from build123d import *

# Parameters (mm, degrees)
SKETCH1_W           = 93.58
SKETCH1_H           = 68.18
BOSS_EXTRUDE1_DEPTH = 5
SKETCH1_12_W        = 73.58
SKETCH1_12_H        = 48.18
CUT_EXTRUDE2_DEPTH  = 59.107075301
FILLET1_R           = 5
FILLET2_R           = 5
SKETCH1_13_R        = 2
CUT_EXTRUDE3_DEPTH  = 59.107075301
SKETCH2_W           = 50.18
SKETCH2_H           = 1.1
CUT_EXTRUDE4_DEPTH  = 88.58


with BuildPart() as part:
    # Sketch1 → Boss-Extrude1 (new body)
    with BuildSketch(Plane(origin=(0, 0, 0), x_dir=(1, 0, 0), z_dir=(0, 1, 0))):
        Rectangle(SKETCH1_W, SKETCH1_H)
    extrude(amount=BOSS_EXTRUDE1_DEPTH)

    # Sketch1<12> → Cut-Extrude2 (cut, through all)
    with BuildSketch(Plane(origin=(0, 0, 0), x_dir=(1, 0, 0), z_dir=(0, 1, 0))):
        Rectangle(SKETCH1_12_W, SKETCH1_12_H)
    extrude(amount=CUT_EXTRUDE2_DEPTH, mode=Mode.SUBTRACT)

    # Fillet1
    fillet1_edges = [part.edges().sort_by_distance(p)[0] for p in [
        (-46.79, 2.5, 34.09),
        (-46.79, 2.5, -34.09),
        (46.79, 2.5, -34.09),
        (46.79, 2.5, 34.09),
    ]]
    fillet(fillet1_edges, radius=FILLET1_R)

    # Fillet2
    fillet2_edges = [part.edges().sort_by_distance(p)[0] for p in [
        (-36.79, 2.5, -24.09),
        (-36.79, 2.5, 24.09),
        (36.79, 2.5, 24.09),
        (36.79, 2.5, -24.09),
    ]]
    fillet(fillet2_edges, radius=FILLET2_R)

    # Sketch1<13> → Cut-Extrude3 (cut, through all)
    with BuildSketch(Plane(origin=(0, 0, 0), x_dir=(1, 0, 0), z_dir=(0, 1, 0))):
        with Locations(Location((-41.79, 29.09, 0), (0, 0, 270))):
            Circle(SKETCH1_13_R)
        with Locations(Location((41.79, 29.09, 0), (0, 0, 90))):
            Circle(SKETCH1_13_R)
        with Locations(Location((41.79, -29.09, 0), (0, 0, 270))):
            Circle(SKETCH1_13_R)
        with Locations(Location((-41.79, -29.09, 0), (0, 0, 90))):
            Circle(SKETCH1_13_R)
    extrude(amount=CUT_EXTRUDE3_DEPTH, mode=Mode.SUBTRACT)

    # Sketch2 → Cut-Extrude4 (cut)
    with BuildSketch(Plane.ZY.offset(46.79)):
        with Locations((0, 2.5)):
            Rectangle(SKETCH2_W, SKETCH2_H)
    extrude(amount=-CUT_EXTRUDE4_DEPTH, mode=Mode.SUBTRACT)


solid = part.part
Part model, mm, in its own coordinate system. A direction names the side the tool comes from. Give positions to 0.01 mm unless a question says otherwise; leave off trailing zeros. Loops run counter-clockwise (first coordinate to the right, second up) from the corner with the lowest first, then second, coordinate; pieces in that order, holes last. Notation, with made-up numbers: M 28,19.5 L 79,19.5 A34 cw 79,51.5 Z; hole C 51,-26.5 d4. An arc over 180 degrees is marked long. Put each result on its own line as item: value. Start each with the question number.
1) Pull direction X, two halves, no side cores. Call faces 3 (the flat face through (-19.1, 3.05, -24.3)), 4 (the cylindrical face through (35.29, 0.99, 22.66)), 5 (the cylindrical face through (-45.36, 2.54, 32.59)), 6 (the cylindrical face through (-43.742, 2.465, -29.524)): +X half, -X half, draft (parallel to the pull), parting line (faces both ways), or undercut.
2) Flat gauge pins, fed straight in: pin 1 (3.5 mm diameter, centred on x = 41.79, z = -29.09, fed in from +Y); pin 2 (5 mm diameter, centred on x = -41.79, z = 29.09, fed in from -Y); pin 3 (0.9 mm diameter, centred on y = 2.5, z = -7.5, fed in from -X). Where does each tip first touch, or does it go through?
3) Saw through at D-D (z = 23). List the corners of the cut face in (x, y), then the cut area to 3 significant figures.
4) Saw through at A-A (x = 2.5). List the corners of the cut face in (y, z).
5) Probe probe 1 along X at (y, z) = (2.35, -29.09); probe 2 along Z at (x, y) = (-41.79, 1.3); probe 3 along Z at (x, y) = (-33, 2.5). List the from-to ranges inside material, lowest first.
6) 3-axis set-ups, long thin cutter, end or side, ignore diameter. For faces 1 (the flat face through (-1, 2, -34.09)), 2 (the flat face through (0, 1, -24.09)): which of +Z, -Z, +X, -X, +Y, -Y reach the whole face in a straight line?
7) Saw through at C-C (y = 4.15). List the corners of the cut face in (x, z).
8) Saw through at B-B (z = -8). List the corners of the cut face in (x, y), then the cut area to 3 significant figures.
Numbers:
1. face 3: draft
1. face 4: undercut
1. face 5: -X half
1. face 6: undercut
2. pin 1: through
2. pin 2: y = 0
2. pin 3: x = 41.79
3. outline: M -46.79,0 L -34.91,0 L -34.91,1.95 L -46.79,1.95 Z; M -46.79,3.05 L -34.91,3.05 L -34.91,5 L -46.79,5 Z; M 34.91,0 L 46.79,0 L 46.79,5 L 34.91,5 L 34.91,3.05 L 41.79,3.05 L 41.79,1.95 L 34.91,1.95 Z
3. area: 98.2 mm^2
4. outline: M 0,-34.09 L 5,-34.09 L 5,-24.09 L 3.05,-24.09 L 3.05,-25.09 L 1.95,-25.09 L 1.95,-24.09 L 0,-24.09 Z; M 0,24.09 L 1.95,24.09 L 1.95,25.09 L 3.05,25.09 L 3.05,24.09 L 5,24.09 L 5,34.09 L 0,34.09 Z
5. probe 1: -46.79 to -43.79, -39.79 to 39.79, 43.79 to 46.79
5. probe 2: -34.09 to -31.09, -27.09 to 27.09, 31.09 to 34.09
5. probe 3: -34.09 to -25.09, 25.09 to 34.09
6. face 1: -Z, +X, -X, +Y, -Y
6. face 2: +Y, -Y
7. outline: M -46.79,-29.09 A5 ccw -41.79,-34.09 L 41.79,-34.09 A5 ccw 46.79,-29.09 L 46.79,29.09 A5 ccw 41.79,34.09 L -41.79,34.09 A5 ccw -46.79,29.09 Z; hole C -41.79,-29.09 d4; hole C -41.79,29.09 d4; hole M -36.79,-19.09 A5 ccw -31.79,-24.09 L 31.79,-24.09 A5 ccw 36.79,-19.09 L 36.79,19.09 A5 ccw 31.79,24.09 L -31.79,24.09 A5 ccw -36.79,19.09 Z; hole C 41.79,-29.09 d4; hole C 41.79,29.09 d4
8. outline: M -46.79,0 L -36.79,0 L -36.79,1.95 L -46.79,1.95 Z; M -46.79,3.05 L -36.79,3.05 L -36.79,5 L -46.79,5 Z; M 36.79,0 L 46.79,0 L 46.79,5 L 36.79,5 L 36.79,3.05 L 41.79,3.05 L 41.79,1.95 L 36.79,1.95 Z
8. area: 83.5 mm^2
